The model under review builds one solid part; all positions refer to its coordinate system, in mm. Face numbers are marked on the shaded views. A direction names the side the tool comes from. Coordinates: 2 decimals unless noted, no trailing zeros. Order: outer loops, then holes, each group sorted by start corner. A loop starts at its lowest first (then second) coordinate and runs counter-clockwise, first axis right, second up. Notation, with made-up numbers: M -4,78 L 47,78 A30 ccw 47,104 Z; hole C 18.5,53 d8. An arc over 180 degrees is marked long. Answer in a Markdown table with one row per item.
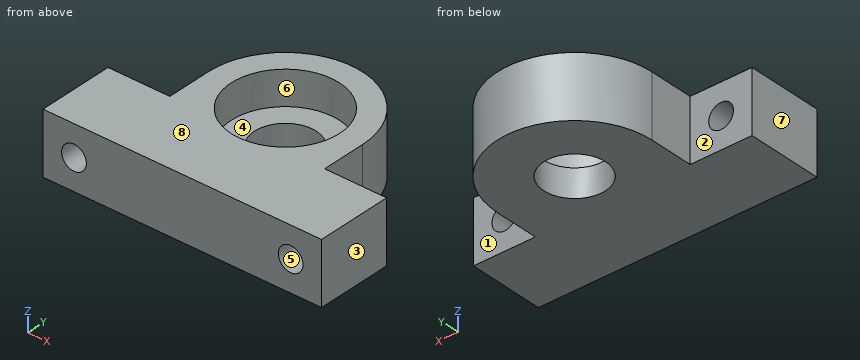
from build123d import *

# Parameters (mm, degrees)
SKETCH1_R           = 25
SKETCH1_R_2         = 17.5
BOSS_EXTRUDE1_DEPTH = 20
BOSS_EXTRUDE2_START = -20
BOSS_EXTRUDE2_DEPTH = 20
SKETCH3_R           = 20
SKETCH3_R_2         = 10
BOSS_EXTRUDE3_DEPTH = 9
SKETCH4_R           = 4
CUT_EXTRUDE1_DEPTH  = 30


with BuildPart() as part:
    # Sketch1 → Boss-Extrude1 (new body)
    with BuildSketch(Plane.XY):
        Circle(SKETCH1_R)
        Circle(SKETCH1_R_2, mode=Mode.SUBTRACT)
    extrude(amount=BOSS_EXTRUDE1_DEPTH)

    # Sketch2 → Boss-Extrude2 (add)
    with BuildSketch(Plane.XY.offset(20).offset(BOSS_EXTRUDE2_START)):
        with BuildLine():
            Line((25, 0), (25, -14.411258269))
            Line((25, -14.411258269), (45, -14.411258269))
            Line((45, -14.411258269), (45, -38.991258269))
            Line((45, -38.991258269), (-45, -38.991258269))
            Line((-45, -38.991258269), (-45, -14.411258269))
            Line((-45, -14.411258269), (-25, -14.411258269))
            Line((-25, -14.411258269), (-25, 0))
            ThreePointArc((-25, 0), (0, -25), (25, 0))
        make_face()
    extrude(amount=BOSS_EXTRUDE2_DEPTH)

    # Sketch3 → Boss-Extrude3 (add)
    with BuildSketch(Plane(origin=(0, 0, 0), x_dir=(-1, 0, 0), z_dir=(0, 0, -1))):
        Circle(SKETCH3_R)
        Circle(SKETCH3_R_2, mode=Mode.SUBTRACT)
    extrude(amount=-BOSS_EXTRUDE3_DEPTH)

    # Sketch4 → Cut-Extrude1 (cut)
    with BuildSketch(Plane(origin=(0, -14.411258269, 0), x_dir=(1, 0, 0), z_dir=(0, 1, 0))):
        with Locations(Location((35, -10, 0), (0, 0, 270))):
            Circle(SKETCH4_R)
        with Locations((-35, -10)):
            Circle(SKETCH4_R)
    extrude(amount=-CUT_EXTRUDE1_DEPTH, mode=Mode.SUBTRACT)


solid = part.part
(1) Insertion check: P1, Ø4, axis at y = 14.5, z = 15, coming from the +X side; P2, Ø2, axis at y = -6.5, z = 13, coming from the -X side; P3, Ø7, axis at y = -4.5, z = 7, coming from the +X side. Each pin has a flat end and moves straight along its axis. Give the tip position at first contact, or say it passes through.
Report:
| item | result |
|---|---|
| P1 | x = 21.65 |
| P2 | x = -25 |
| P3 | x = 25 |
(2) To check wall thickness, follow line 1 (X direction, y = -29.5, z = 10); line 2 (X direction, y = -15, z = 6.5); line 3 (Y direction, x = 0, z = 5). State the ranges of each line that lie inside material, in increasing order. Write a range as [from, to].
Report:
| item | result |
|---|---|
| line 1 | [-45, -39], [-31, 31], [39, 45] |
| line 2 | [-45, -36.94], [-33.06, 33.06], [36.94, 45] |
| line 3 | [-38.99, -10], [10, 25] |
(3) Take a section at A-A (z = 10). Write out the cut boundary in (x, y).
Report:
| item | result |
|---|---|
| outline | M -45,-38.99 L -39,-38.99 L -39,-14.41 L -45,-14.41 Z; M -31,-38.99 L 31,-38.99 L 31,-14.41 L 25,-14.41 L 25,0 A25 ccw -25,0 L -25,-14.41 L -31,-14.41 Z; M 39,-38.99 L 45,-38.99 L 45,-14.41 L 39,-14.41 Z; hole C 0,0 d35 |
(4) Take a section at C-C (y = -26). Write out the cut boundary in (x, z).
Report:
| item | result |
|---|---|
| outline | M -45,0 L 45,0 L 45,20 L -45,20 Z; hole C -35,10 d8; hole C 35,10 d8 |
(5) Take a section at B-B (x = 0). Write out the cut boundary in (y, z).
Report:
| item | result |
|---|---|
| outline | M -38.99,0 L -10,0 L -10,9 L -17.5,9 L -17.5,20 L -38.99,20 Z; M 10,0 L 25,0 L 25,20 L 17.5,20 L 17.5,9 L 10,9 Z |
(6) Machinability: for the marked faces 1, 2, 3 and 4, which of the approach directions +Z, -Z, +X, -X, +Y, -Y give a long, thin tool a straight path to every point of the face, cutting with its end or side? Answer none if there is none.
Report:
| item | result |
|---|---|
| face 1 | +Z, -Z, +X, +Y |
| face 2 | +Z, -Z, -X, +Y |
| face 3 | +Z, -Z, +X, +Y, -Y |
| face 4 | +Z |
(7) The part is to be moulded in two halves that separate along X. For the marked faces 5, 6, 7 and 8, say which applies: +X half, -X half, draft (parallel to the pull), parting line (faces both ways), or undercut.
Report:
| item | result |
|---|---|
| face 5 | undercut |
| face 6 | undercut |
| face 7 | -X half |
| face 8 | draft |
(8) Take a section at D-D (z = 4.75). Write out the cut boundary in (x, y).
Report:
| item | result |
|---|---|
| outline | M -45,-38.99 L 45,-38.99 L 45,-14.41 L 25,-14.41 L 25,0 A25 ccw -25,0 L -25,-14.41 L -45,-14.41 Z; hole C 0,0 d20 |
